from build123d import *

# Parameters (mm, degrees)
SKETCH1_W            = 202
SKETCH1_H            = 133
BOSS_EXTRUDE1_DEPTH  = 69
SKETCH2_W            = 18.5
SKETCH2_H            = 18.5
BOSS_EXTRUDE2_DEPTH  = 3.5
M6_CLEARANCE_HOLE1_D = 6.6


with BuildPart() as part:
    # Sketch1 → Boss-Extrude1 (new body)
    with BuildSketch(Plane(origin=(0, 0, 0), x_dir=(1, 0, 0), z_dir=(0, 1, 0))):
        with Locations((101, 66.5)):
            Rectangle(SKETCH1_W, SKETCH1_H)
    extrude(amount=BOSS_EXTRUDE1_DEPTH)

    # Sketch2 → Boss-Extrude2 (add)
    with BuildSketch(Plane(origin=(0, 0, 0), x_dir=(1, 0, 0), z_dir=(0, 1, 0))):
        with Locations((-9.25, 123.75)):
            Rectangle(SKETCH2_W, SKETCH2_H)
        with Locations((-9.25, 9.25)):
            Rectangle(SKETCH2_W, SKETCH2_H)
        with Locations((211.25, 9.25)):
            Rectangle(SKETCH2_W, SKETCH2_H)
        with Locations((211.25, 123.75)):
            Rectangle(SKETCH2_W, SKETCH2_H)
    extrude(amount=BOSS_EXTRUDE2_DEPTH)

    # M6 Clearance Hole1 (through all)
    with Locations(Plane(origin=(0, 3.5, 0), x_dir=(1, 0, 0), z_dir=(0, 1, 0))):
        with Locations((-10, 123.75), (-10, 9.25), (212, 9.25), (212, 123.75)):
            Hole(M6_CLEARANCE_HOLE1_D / 2)


solid = part.part
CAD build for the part. Positions are in the model's coordinates, mm. A direction names the side the tool comes from. Give positions to 0.01 mm unless a question says otherwise; leave off trailing zeros. Loops run counter-clockwise (first coordinate to the right, second up) from the corner with the lowest first, then second, coordinate; pieces in that order, holes last. Notation, with made-up numbers: M 13.5,-14 L 49.5,-14 A12 ccw 49.5,-3 Z; hole C 85,30 d5. An arc over 180 degrees is marked long. Answer in a Markdown table with one row per item. Add a question column.
Item 1: Probe probe 1 along Z at (x, y) = (-10, 1); probe 2 along X at (y, z) = (1.9, -9.25); probe 3 along X at (y, z) = (64.5, -89). List the from-to ranges inside material, lowest first.
Item 2: Band-saw the part on C-C on y = 64. Give the cut face in (x, z).
Item 3: Tool access for faces 3 (the face through (209, 3.5, -7)), 4 (the face through (-7, 3.5, -11)), 5 (the face through (99, 0, -67)): list every direction of +Z, -Z, +X, -X, +Y, -Y with a clear straight run to the whole face (end or side of a thin tool).
Item 4: Drop flat-ended pins along their axis: P1, Ø10.5, axis at x = -10, z = -123.75, coming from the +Y side; P2, Ø5, axis at y = 57.5, z = -79.5, coming from the -X side; P3, Ø5, axis at y = 13, z = -21.5, coming from the +X side; P4, Ø5.5, axis at x = -10, z = -9.25, coming from the +Y side. Give the stop position or say it passes through.
Item 5: Band-saw the part on B-B on z = -123.75. Give the cut face in (x, y).
Item 6: Mould opens along X. For faces 1 (the face through (212.72, 1.73, -120.53)), 2 (the face through (209, 3.5, -122)) say: +X half, -X half, draft (parallel to the pull), parting line (faces both ways), or undercut.
Item 7: Band-saw the part on A-A on x = -10. Give the cut face in (y, z).
Item 8: Band-saw the part on D-D on z = -81.5. Give the cut face in (x, y), then the cut area to 3 significant figures.
Reply:
| question | item | result |
|---|---|---|
| 1 | probe 1 | z = -133 to -127.05, -120.45 to -114.5, -18.5 to -12.55, -5.95 to 0 |
| 1 | probe 2 | x = -18.5 to -13.3, -6.7 to 208.7, 215.3 to 220.5 |
| 1 | probe 3 | x = 0 to 202 |
| 2 | outline | M 0,-133 L 202,-133 L 202,0 L 0,0 Z |
| 3 | face 3 | +Z, -Z, +X, +Y |
| 3 | face 4 | +Z, -Z, -X, +Y |
| 3 | face 5 | +Z, -Z, +X, -X, -Y |
| 4 | P1 | stops at y = 3.5 |
| 4 | P2 | stops at x = 0 |
| 4 | P3 | stops at x = 202 |
| 4 | P4 | passes through |
| 5 | outline | M -18.5,0 L -13.3,0 L -13.3,3.5 L -18.5,3.5 Z; M -6.7,0 L 208.7,0 L 208.7,3.5 L 202,3.5 L 202,69 L 0,69 L 0,3.5 L -6.7,3.5 Z; M 215.3,0 L 220.5,0 L 220.5,3.5 L 215.3,3.5 Z |
| 6 | face 1 | undercut |
| 6 | face 2 | draft |
| 7 | outline | M 0,-133 L 3.5,-133 L 3.5,-127.05 L 0,-127.05 Z; M 0,-120.45 L 3.5,-120.45 L 3.5,-114.5 L 0,-114.5 Z; M 0,-18.5 L 3.5,-18.5 L 3.5,-12.55 L 0,-12.55 Z; M 0,-5.95 L 3.5,-5.95 L 3.5,0 L 0,0 Z |
| 8 | outline | M 0,0 L 202,0 L 202,69 L 0,69 Z |
| 8 | area | 13,900 mm^2 |
